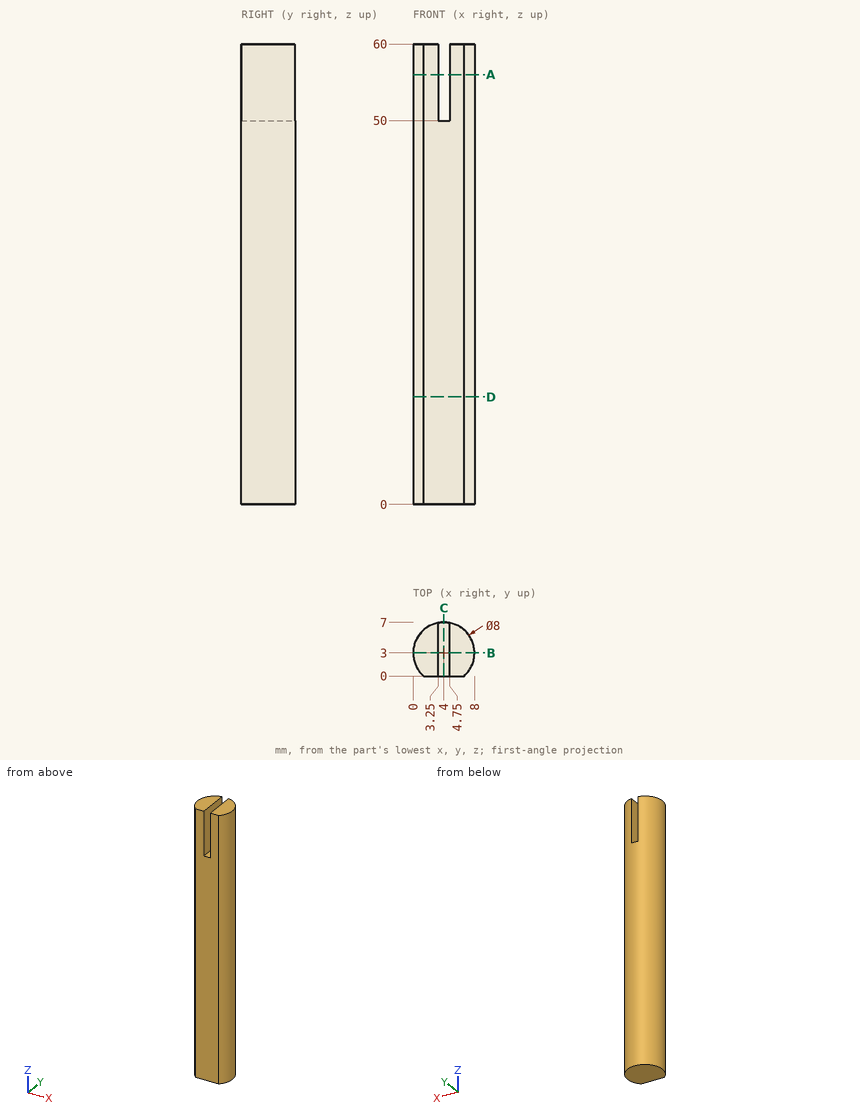
Input: dimensioned drawing with shaded views. Units: mm. Origin: part minimum x, y, z. Round coordinates to 2 decimals unless told otherwise and drop trailing zeros. Order: outer loops, then holes, each group sorted by start corner. A loop starts at its lowest first (then second) coordinate and runs counter-clockwise, first axis right, second up.
1. Cut plane B-B, the plane y = 3. Output: boundary loops of the cut face in (x, z), then the cut area to 3 significant figures.
The answers:
outline: (0, 0) - (8, 0) - (8, 60) - (4.75, 60) - (4.75, 50) - (3.25, 50) - (3.25, 60) - (0, 60) - close
area: 465 mm2
2. Pin query (flat end, axial travel): P1, Ø1.2, axis at x = 4, y = 2, coming from the +Z side; P2, Ø1, axis at x = 7, z = 37.5, coming from the +Y side; P3, Ø2, axis at y = 1.5, z = 12.5, coming from the +X side. Return the tip coordinate at first contact, or that it passes through.
The answers:
P1: stops at z = 50
P2: stops at y = 6.12
P3: stops at x = 7.97
3. Material intervals for line 1 (Z direction, x = 4.5, y = 1); line 2 (X direction, y = 3.25, z = 19.5); line 3 (X direction, y = 1.25, z = 52), sorted ascending.
The answers:
line 1: z = 0 to 50
line 2: x = 0.01 to 7.99
line 3: x = 0.4 to 3.25, 4.75 to 7.6
4. Cut plane A-A, the plane z = 56. Output: boundary loops of the cut face in (x, y), then the cut area to 3 significant figures.
The answers:
outline: (1.35, 0) - (3.25, 0) - (3.25, 6.93) arc R4 ccw to start; (4.75, 0) - (6.65, 0) arc R4 ccw to (4.75, 6.93) - close
area: 36.2 mm2
5. Cut plane C-C, the plane x = 4. Output: boundary loops of the cut face in (y, z).
The answers:
outline: (0, 0) - (7, 0) - (7, 50) - (0, 50) - close
6. Cut plane D-D, the plane z = 14. Output: boundary loops of the cut face in (x, y), then the cut area to 3 significant figures.
The answers:
outline: (1.35, 0) - (6.65, 0) arc R4 ccw (long way) to start
area: 46.6 mm2
